Can you work these out from the model? Positions are in its coordinate system, mm. Face numbers are marked on the shaded views. A direction names the side the tool comes from. Give positions to 0.01 mm unless a question says otherwise; leave off trailing zeros. Write each loop counter-clockwise with the first axis right and the second up, starting at its lowest first coordinate (ties: lowest second). Pieces come first, ordered by that corner, then holes.
```python
from build123d import *

# Parameters (mm, degrees)
ESBO_O1_OUTSIDE_W     = 192.158
ESBO_O1_OUTSIDE_H     = 192.158
CORTE_EXTRUS_O1_DEPTH = 108.596468344
CORTE_EXTRUS_O2_START = -4
ESBO_O3_W             = 70
ESBO_O3_H             = 70
CORTE_EXTRUS_O2_DEPTH = 90.21748763
FILETE1_R             = 15
ESBO_O4_W             = 127
ESBO_O4_H             = 2
CORTE_EXTRUS_O4_DEPTH = 92.320862119
ESBO_O5_W             = 6
ESBO_O5_H             = 2
CORTE_EXTRUS_O5_DEPTH = 92.320862119
ESBO_O6_R             = 1.5
CORTE_EXTRUS_O7_DEPTH = 93.131236882
CORTE_EXTRUS_O8_START = -4
CORTE_EXTRUS_O8_DEPTH = 89.131236882


with BuildPart() as part:
    # Esboço2 → Revolução1 (revolve)
    with BuildSketch(Plane(origin=(0, 0, 0), x_dir=(0, 0, -1), z_dir=(1, 0, 0)), mode=Mode.PRIVATE) as revolu_o1_sk:
        with BuildLine():
            Line((0, 74), (4, 74))
            ThreePointArc((4, 74), (19.648353468, 38.461019227), (25, 0))
            Line((25, 0), (0, 0))
            Line((0, 0), (0, 74))
        make_face()
    revolve(revolu_o1_sk.sketch.rotate(Axis((0, 0, 0), (0, 0, -1)), 90), axis=Axis((0, 0, 0), (0, 0, -1)))

    # Esboço1 outside → Corte-extrusão1 (cut, through all)
    with BuildSketch(Plane.XY):
        Rectangle(ESBO_O1_OUTSIDE_W, ESBO_O1_OUTSIDE_H)
        Polygon((63.5, 26.302561211), (26.302561211, 63.5), (-26.302561211, 63.5), (-63.5, 26.302561211), (-63.5, -26.302561211), (-26.302561211, -63.5), (26.302561211, -63.5), (63.5, -26.302561211), align=None, mode=Mode.SUBTRACT)
    extrude(amount=-CORTE_EXTRUS_O1_DEPTH, mode=Mode.SUBTRACT)

    # Esboço3 → Corte-extrusão2 (cut, through all)
    with BuildSketch(Plane.XY.offset(CORTE_EXTRUS_O2_START)):
        Rectangle(ESBO_O3_W, ESBO_O3_H)
    extrude(amount=-CORTE_EXTRUS_O2_DEPTH, mode=Mode.SUBTRACT)

    # Filete1
    filete1_edges = [part.edges().sort_by_distance(p)[0] for p in [
        (35, 35, -10.009206795),
        (35, -35, -10.009206795),
        (-35, -35, -10.009206795),
        (-35, 35, -10.009206795),
    ]]
    fillet(filete1_edges, radius=FILETE1_R)

    # Esboço4 → Corte-extrusão4 (cut, through all)
    with BuildSketch(Plane.XY.offset(-4)):
        with Locations((0, 25.302561211)):
            Rectangle(ESBO_O4_W, ESBO_O4_H)
    extrude(amount=-CORTE_EXTRUS_O4_DEPTH, mode=Mode.SUBTRACT)

    # Esboço5 → Corte-extrusão5 (cut, through all)
    with BuildSketch(Plane(origin=(0, 0, -4), x_dir=(-1, 0, 0), z_dir=(0, 0, -1))):
        with Locations((-60.5, 25.302561211)):
            Rectangle(ESBO_O5_W, ESBO_O5_H)
        with Locations((60.5, 25.302561211)):
            Rectangle(ESBO_O5_W, ESBO_O5_H)
    extrude(amount=-CORTE_EXTRUS_O5_DEPTH, mode=Mode.SUBTRACT)

    # Esboço6 → Corte-extrusão7 (cut, through all)
    with BuildSketch(Plane.XY):
        with Locations((42.072853481, -42.072853481)):
            Circle(ESBO_O6_R)
        with Locations((-42.072853481, -42.072853481)):
            Circle(ESBO_O6_R)
        with Locations((-42.072853481, 42.072853481)):
            Circle(ESBO_O6_R)
        with Locations((42.072853481, 42.072853481)):
            Circle(ESBO_O6_R)
    extrude(amount=-CORTE_EXTRUS_O7_DEPTH, mode=Mode.SUBTRACT)

    # Esboço7 → Corte-extrusão8 (cut, through all)
    with BuildSketch(Plane.XY.offset(CORTE_EXTRUS_O8_START)):
        with BuildLine():
            Line((42.603183566, 47.199377644), (39.774756442, 44.370950519))
            ThreePointArc((39.774756442, 44.370950519), (39.774756442, 39.774756442), (44.370950519, 39.774756442))
            Line((44.370950519, 39.774756442), (47.199377644, 42.603183566))
            Line((47.199377644, 42.603183566), (42.603183566, 47.199377644))
        make_face()
        with BuildLine():
            Line((-47.199377644, 42.603183566), (-44.370950519, 39.774756442))
            ThreePointArc((-44.370950519, 39.774756442), (-39.774756442, 39.774756442), (-39.774756442, 44.370950519))
            Line((-39.774756442, 44.370950519), (-42.603183566, 47.199377644))
            Line((-42.603183566, 47.199377644), (-47.199377644, 42.603183566))
        make_face()
        with BuildLine():
            Line((47.199377644, -42.603183566), (44.370950519, -39.774756442))
            ThreePointArc((44.370950519, -39.774756442), (39.774756442, -39.774756442), (39.774756442, -44.370950519))
            Line((39.774756442, -44.370950519), (42.603183566, -47.199377644))
            Line((42.603183566, -47.199377644), (47.199377644, -42.603183566))
        make_face()
        with BuildLine():
            Line((-42.603183566, -47.199377644), (-39.774756442, -44.370950519))
            ThreePointArc((-39.774756442, -44.370950519), (-39.774756442, -39.774756442), (-44.370950519, -39.774756442))
            Line((-44.370950519, -39.774756442), (-47.199377644, -42.603183566))
            Line((-47.199377644, -42.603183566), (-42.603183566, -47.199377644))
        make_face()
    extrude(amount=-CORTE_EXTRUS_O8_DEPTH, mode=Mode.SUBTRACT)


solid = part.part
```
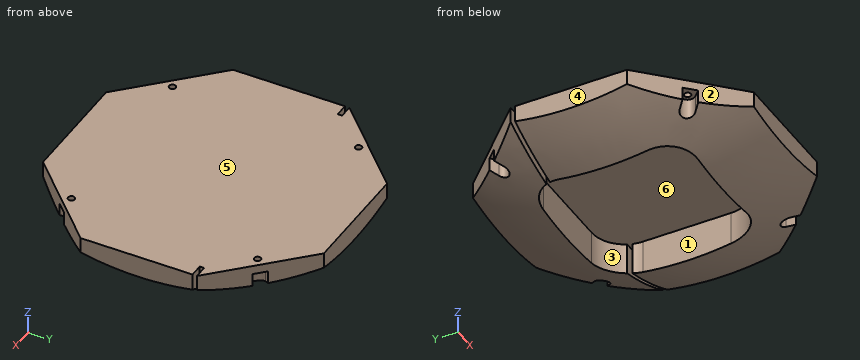
1) Suppose I cut it at C-C on y = 12. Write out the boundary of the cut face in (x, z), plus the area to 3 significant figures.
Values follow:
outline: (-63.5, -9.3) arc R140.37 ccw to (-35, -20.05) - (-35, -4) - (35, -4) - (35, -20.05) arc R140.37 ccw to (63.5, -9.3) - (63.5, 0) - (-63.5, 0) - close
area: 1,150 mm2
2) If we mould it in two halves opening along Y, with no side actions, what happens to the marked faces 1, 2, 3 and 4? For each: +Y half, -Y half, draft (parallel to the pull), parting line (faces both ways), or undercut.
Values follow:
face 1: undercut
face 2: -Y half
face 3: undercut
face 4: draft
3) Suppose I cut it at D-D on y = -52.5. Write out the boundary of the cut face in (x, z).
Values follow:
outline: (-37.3, -9.42) arc R130.73 ccw to (37.3, -9.42) - (37.3, 0) - (-37.3, 0) - close
4) For pin 1 Ø1.5 at (y, z) = (1, -14) entering from -X; pin 2 Ø1.5 at (x, z) = (-50.5, -7) entering from -Y; pin 3 Ø5 at (y, z) = (6.5, -13.5) entering from -X; pin 4 Ø2.5 at (x, y) = (-42.07, -42.07) entering from -Z, each with a flat end and sliding along its axis, tell me the tip position at first contact or that it passes through.
Values follow:
pin 1: stops at x = -56.32
pin 2: stops at y = -40.05
pin 3: stops at x = -60.89
pin 4: passes through
5) Suppose I cut it at B-B on x = -9. Write out the boundary of the cut face in (y, z), plus the area to 3 significant figures.
Values follow:
outline: (-63.5, -9.56) arc R140.59 ccw to (-35, -20.29) - (-35, -4) - (35, -4) - (35, -20.29) arc R140.59 ccw to (63.5, -9.56) - (63.5, 0) - (-63.5, 0) - close
area: 1,160 mm2
6) Suppose I cut it at A-A on z = -1.5. Write out the boundary of the cut face in (x, y).
Values follow:
outline: (-63.5, -26.3) - (-26.3, -63.5) - (26.3, -63.5) - (63.5, -26.3) - (63.5, 24.3) - (57.5, 24.3) - (57.5, 26.3) - (63.5, 26.3) - (26.3, 63.5) - (-26.3, 63.5) - (-63.5, 26.3) - (-57.5, 26.3) - (-57.5, 24.3) - (-63.5, 24.3) - close; hole circle Ø3 at (-42.07, -42.07); hole circle Ø3 at (-42.07, 42.07); hole circle Ø3 at (42.07, -42.07); hole circle Ø3 at (42.07, 42.07)
7) Please list where these lines run through material, in increasing order: L1, parallel to Y at x = -8, z = -4.5; L2, parallel to Z at x = -8, y = 22.5; L3, parallel to X at y = -13, z = -9.5.
Values follow:
L1: y = -63.5 to -35, 35 to 63.5
L2: z = -4 to 0
L3: x = -62.91 to -35, 35 to 62.91
8) For the marked faces 5 and 6, which set-ups out of +Z, -Z, +X, -X, +Y, -Y let a thin tool reach every point of the face, with its end or its side?
Values follow:
face 5: +Z, +X, -X, +Y, -Y
face 6: -Z
